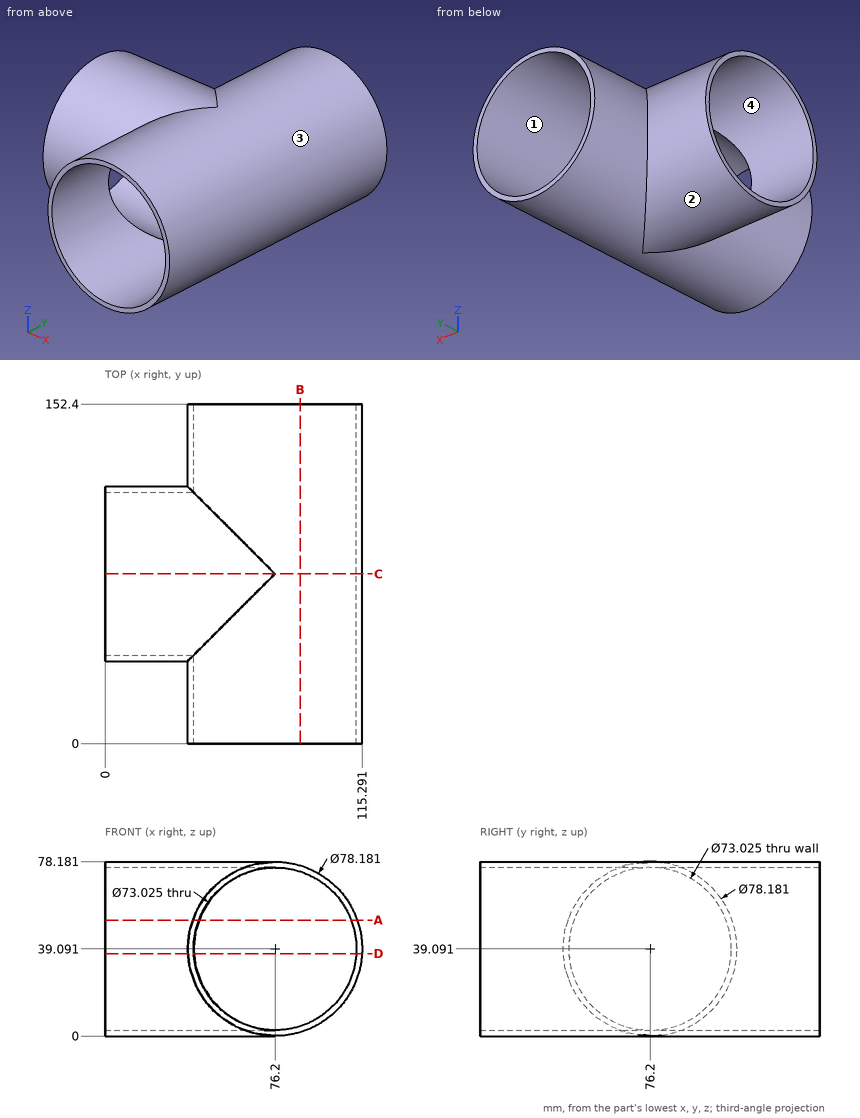
Design review of the part shown in the three views and the two pictorial views. Dimensions are in mm from the part's minimum x, y and z. A direction names the side the tool comes from. Round coordinates to 2 decimals unless told otherwise and drop trailing zeros. Write each loop counter-clockwise with the first axis right and the second up, starting at its lowest first coordinate (ties: lowest second). Pieces come first, ordered by that corner, then holes. Notation, with made-up numbers: (64, 64.25) - (74, 64.25) arc R22 ccw to (74, 100.25) - close; hole circle Ø8 at (33.5, -33.5). An arc over 180 degrees is marked (long way). Answer as CSV lines item,"result". Start each with the question number.
(1) Mouldability with a two-part tool opening along Z and no side actions: class the marked faces 1 and 2 as +Z half, -Z half, draft (parallel to the pull), parting line (faces both ways), or undercut.
(2) Add section A-A, the plane z = 52. State the section outline as (x, y) points (1 decimal).
(3) Add section C-C, the plane y = 76.2. State the section outline as (x, z) points (1 decimal).
(4) Add section D-D, the plane z = 37. State the section outline as (x, y) points (1 decimal).
(5) For pin 1 (5 mm diameter, centred on y = 125, z = 70, fed in from -X); pin 2 (5 mm diameter, centred on y = 132, z = 25, fed in from -X); pin 3 (3 mm diameter, centred on x = 29.5, y = 65, fed in from +Z), all flat-tipped, find the tip position at first contact; note any pin that passes through.
(6) Add section B-B, the plane x = 87.5. State the section outline as (y, z) points.
(7) For line 1 (Z direction, x = 76.2, y = 83.5); line 2 (X direction, y = 123.5, z = 27) (1 decimal); line 3 (Z direction, x = 94.5, y = 142) (1 decimal), list the stretches that pass through material, from the lowest coordinate up.
(8) Machinability: for the marked faces 3 and 4, which of the approach directions +Z, -Z, +X, -X, +Y, -Y give a long, thin tool a straight path to every point of the face, cutting with its end or side? Answer none if there is none.
From the geometry:
1,face 1,"undercut"
1,face 2,"parting line"
2,outline,"(0, 39.3) - (39.3, 39.3) - (39.3, 0) - (42, 0) - (42, 42) - (0, 42) - close; (0, 110.4) - (42, 110.4) - (42, 152.4) - (39.3, 152.4) - (39.3, 113.1) - (0, 113.1) - close; (110.4, 0) - (113.1, 0) - (113.1, 152.4) - (110.4, 152.4) - close"
3,outline,"(0, 0) - (76.2, 0) arc R39.1 ccw to (76.2, 78.2) - (0, 78.2) - (0, 75.6) - (76.2, 75.6) arc R36.5 cw to (76.2, 2.6) - (0, 2.6) - close"
4,outline,"(0, 37.2) - (37.2, 37.2) - (37.2, 0) - (39.7, 0) - (39.7, 39.7) - (0, 39.7) - close; (0, 112.7) - (39.7, 112.7) - (39.7, 152.4) - (37.2, 152.4) - (37.2, 115.2) - (0, 115.2) - close; (112.7, 0) - (115.2, 0) - (115.2, 152.4) - (112.7, 152.4) - close"
5,pin 1,"stops at x = 49.35"
5,pin 2,"stops at x = 38.87"
5,pin 3,"stops at z = 76.96"
6,outline,"(0, 1.67) - (152.4, 1.67) - (152.4, 4.37) - (0, 4.37) - close; (0, 73.81) - (152.4, 73.81) - (152.4, 76.51) - (0, 76.51) - close"
7,line 1,"z = 0 to 2.58, 75.6 to 78.18"
7,line 2,"x = 39 to 41.7, 110.7 to 113.4"
7,line 3,"z = 4.5 to 7.5, 70.7 to 73.6"
8,face 3,"none"
8,face 4,"-X"
